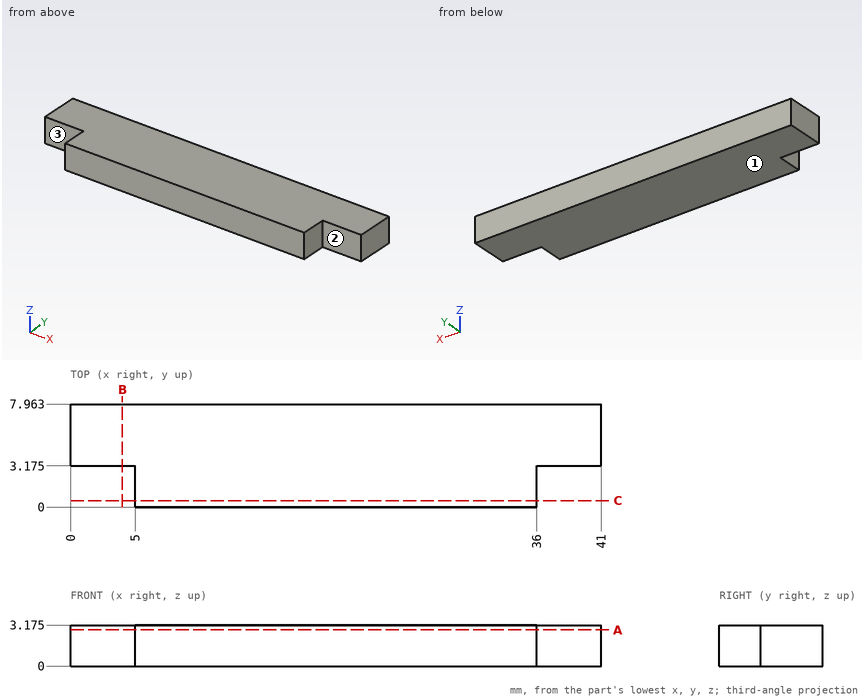
The drawing under review shows one solid part. Ordinate dimensions are in mm from its lowest x, y, z. A direction names the side the tool comes from. Round coordinates to 2 decimals unless told otherwise and drop trailing zeros. Loops run counter-clockwise (first coordinate to the right, second up) from the corner with the lowest first, then second, coordinate; pieces in that order, holes last. Notation, with made-up numbers: (-12, 26.25) -> (-7, 26.25) arc R36 cw to (-7, 65.25) -> close; hole circle Ø6 at (-2, 16). An arc over 180 degrees is marked (long way). One line per question, with ' | ' between items. Start each with the question number.
Item 1: Add section A-A, the plane z = 2.8. Write out the cut boundary in (x, y) (3 decimals), then the cut area to 3 significant figures.
Item 2: Add section B-B, the plane x = 4. Write out the cut boundary in (y, z) (3 decimals).
Item 3: Wall thickness on line 1 along X through (y, z) = (0.5, 0.55); line 2 along Y through (x, z) = (4.5, 0.6) (3 decimals): over which ranges is each line inside the solid? List them lowest first. Write a range as [from, to].
Item 4: Machinability: for the marked faces 1, 2 and 3, which of the approach directions +Z, -Z, +X, -X, +Y, -Y give a long, thin tool a straight path to every point of the face, cutting with its end or side? Answer none if there is none.
Item 5: For pin 1 (4 mm diameter, centred on x = 7.5, y = 6, fed in from -Z); pin 2 (1 mm diameter, centred on x = 1.5, z = 1, fed in from -Y) (3 decimals), all flat-tipped, find the tip position at first contact; note any pin that passes through.
Item 6: Add section C-C, the plane y = 0.5. Write out the cut boundary in (x, z) (3 decimals), then the cut area to 3 significant figures.
Return value:
1) outline: (0, 3.175) -> (5, 3.175) -> (5, 0) -> (36, 0) -> (36, 3.175) -> (41, 3.175) -> (41, 7.963) -> (0, 7.963) -> close | area: 295 mm2
2) outline: (3.175, 0) -> (7.963, 0) -> (7.963, 3.175) -> (3.175, 3.175) -> close
3) line 1: x = [5, 36] | line 2: y = [3.175, 7.963]
4) face 1: -Z, +X, -X, +Y, -Y | face 2: +Z, -Z, +X, -Y | face 3: +Z, -Z, -X, -Y
5) pin 1: stops at z = 0 | pin 2: stops at y = 3.175
6) outline: (5, 0) -> (36, 0) -> (36, 3.175) -> (5, 3.175) -> close | area: 98.4 mm2
